Source: CAD feature listing. Evaluate the final solid. Frame: model axes, mm. Give positions to 0.01 mm unless a question says otherwise; leave off trailing zeros. Loops run counter-clockwise (first coordinate to the right, second up) from the corner with the lowest first, then second, coordinate; pieces in that order, holes last.
from build123d import *

# Parameters (mm, degrees)
SKETCH1_W           = 8
SKETCH1_H           = 10
SKETCH1_R           = 5
SKETCH1_R_2         = 1.5
BOSS_EXTRUDE1_DEPTH = 8
SKETCH2_W           = 4.2
SKETCH2_H           = 4.2
CUT_EXTRUDE1_DEPTH  = 3.5
SKETCH3_W           = 1.5
SKETCH3_H           = 4.2
CUT_EXTRUDE2_DEPTH  = 83.074661132
CHAMFER1_SIZE       = 1
CHAMFER2_SIZE       = 0.5


with BuildPart() as part:
    # Sketch1 → Boss-Extrude1 (new body)
    # profile 1 of 3: a face of its own
    with BuildSketch(Plane(origin=(0, 0, 0), x_dir=(1, 0, 0), z_dir=(0, 1, 0))):
        with BuildLine():
            Line((72, 5), (0, 5))
            ThreePointArc((0, 5), (3.535533906, 3.535533906), (5, 0))
            ThreePointArc((5, 0), (3.535533906, -3.535533906), (0, -5))
            Line((0, -5), (80, -5))
            Line((80, -5), (80, 5))
            Line((80, 5), (72, 5))
        make_face()
    # profile 2 of 3: a face of its own
    with BuildSketch(Plane(origin=(0, 0, 0), x_dir=(1, 0, 0), z_dir=(0, 1, 0))):
        with Locations((76, 10)):
            Rectangle(SKETCH1_W, SKETCH1_H)
    # profile 3 of 3: a face of its own
    with BuildSketch(Plane(origin=(0, 0, 0), x_dir=(1, 0, 0), z_dir=(0, 1, 0))):
        Circle(SKETCH1_R)
        with Locations(Location((0, 0, 0), (0, 0, 270))):
            Circle(SKETCH1_R_2, mode=Mode.SUBTRACT)
    extrude(amount=BOSS_EXTRUDE1_DEPTH)

    # Sketch2 → Cut-Extrude1 (cut)
    with BuildSketch(Plane(origin=(0, 0, -15), x_dir=(-1, 0, 0), z_dir=(0, 0, -1))):
        with Locations((-76, 4)):
            Rectangle(SKETCH2_W, SKETCH2_H)
    extrude(amount=-CUT_EXTRUDE1_DEPTH, mode=Mode.SUBTRACT)

    # Sketch3 → Cut-Extrude2 (cut, through all)
    with BuildSketch(Plane(origin=(0, 0, -11.5), x_dir=(-1, 0, 0), z_dir=(0, 0, -1))):
        with Locations((-77.35, 4)):
            Rectangle(SKETCH3_W, SKETCH3_H)
        with Locations((-74.65, 4)):
            Rectangle(SKETCH3_W, SKETCH3_H)
    extrude(amount=-CUT_EXTRUDE2_DEPTH, mode=Mode.SUBTRACT)

    # Chamfer1
    chamfer1_edges = [part.edges().sort_by_distance(p)[0] for p in [
        (76, 0, -15),
        (80, 0, -5),
        (40, 0, 5),
        (-5, 0, 0),
        (-5, 8, 0),
        (36, 0, -5),
        (40, 8, 5),
        (80, 8, -5),
        (76, 8, -15),
        (72, 8, -10),
        (0, 8, -1.5),
        (36, 8, -5),
        (0, 0, -1.5),
        (72, 0, -10),
    ]]
    chamfer(chamfer1_edges, length=CHAMFER1_SIZE)

    # Chamfer2
    chamfer2_edges = [part.edges().sort_by_distance(p)[0] for p in [
        (78.1, 4, -15),
        (76, 1.9, -15),
        (73.9, 4, -15),
        (76, 6.1, -15),
        (78.1, 4, 5),
        (77.35, 6.1, 5),
        (76.6, 4, 5),
        (77.35, 1.9, 5),
        (73.9, 4, 5),
        (74.65, 1.9, 5),
        (75.4, 4, 5),
        (74.65, 6.1, 5),
    ]]
    chamfer(chamfer2_edges, length=CHAMFER2_SIZE)


solid = part.part
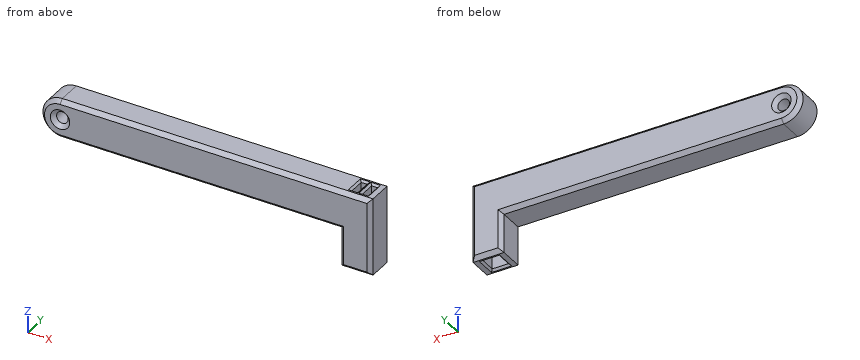
1) Cut plane B-B (z = 0). Return loops of the section in (x, y).
Checks:
outline: (-5, 1) - (-4, 0) - (-2.5, 0) - (-1.5, 1) - (-1.5, 7) - (-2.5, 8) - (-4, 8) - (-5, 7) - close; (1.5, 1) - (2.5, 0) - (79, 0) - (80, 1) - (80, 7) - (79, 8) - (2.5, 8) - (1.5, 7) - close; hole (73.9, 1.9) - (75.4, 1.9) - (75.4, 6.1) - (73.9, 6.1) - close; hole (76.6, 1.9) - (78.1, 1.9) - (78.1, 6.1) - (76.6, 6.1) - close
2) Contact query for flat-ended pins moving along their axis: P1, Ø1.5, axis at x = 21.5, y = 4, coming from the -Z side; P2, Ø3.5, axis at y = 5, z = -2, coming from the -X side; P3, Ø1.3, axis at x = 76, y = 4, coming from the -Z side; P4, Ø2.5, axis at x = 0, z = 0, coming from the +Y side. Output: stop coordinate, or through.
Checks:
P1: stops at z = -5
P2: stops at x = -4.99
P3: stops at z = -11.5
P4: passes through
3) Cut plane D-D (x = 30). Return loops of the section in (y, z).
Checks:
outline: (0, -4) - (1, -5) - (7, -5) - (8, -4) - (8, 4) - (7, 5) - (1, 5) - (0, 4) - close
4) Ray query, probe 1 along X at (y, z) = (2.3, 0); probe 2 along X at (y, z) = (5.5, -11); probe 3 along Y at (x, z) = (74, 3.25). Return the intervals inside material, ascending.
Checks:
probe 1: x = -5 to -1.5, 1.5 to 73.9, 75.4 to 76.6, 78.1 to 80
probe 2: x = 72 to 73.9, 75.4 to 76.6, 78.1 to 80
probe 3: y = 0 to 1.9, 6.1 to 8
5) Cut plane A-A (y = 3.75). Return loops of the section in (x, z).
Checks:
outline: (0, -5) - (72, -5) - (72, -15) - (73.4, -15) - (73.9, -14.5) - (73.9, 4.5) - (73.4, 5) - (0, 5) arc R5 ccw to start; (75.4, -11.5) - (76.6, -11.5) - (76.6, 4.5) - (76.1, 5) - (75.9, 5) - (75.4, 4.5) - close; (78.1, -14.5) - (78.6, -15) - (80, -15) - (80, 5) - (78.6, 5) - (78.1, 4.5) - close; hole circle Ø3 at (0, 0)
6) Cut plane C-C (z = -6.25). Return loops of the section in (x, y).
Checks:
outline: (72, 1) - (73, 0) - (79, 0) - (80, 1) - (80, 7) - (79, 8) - (73, 8) - (72, 7) - close; hole (73.9, 1.9) - (75.4, 1.9) - (75.4, 6.1) - (73.9, 6.1) - close; hole (76.6, 1.9) - (78.1, 1.9) - (78.1, 6.1) - (76.6, 6.1) - close
